Study the drawing (mm; zero at the part's minimum x, y, z) and answer. A direction names the side the tool comes from. Coordinates: 2 decimals unless noted, no trailing zeros. Write each loop counter-clockwise with the first axis right and the second up, starting at its lowest first coordinate (ties: lowest second). Pieces come first, ordered by that corner, then holes. Notation, with made-up numbers: (59, 48.5) -> (104, 48.5) arc R21 ccw to (104, 74.5) -> close; hole circle Ø4 at (41, -18). An arc over 180 degrees is marked (long way). Write each question's results on one line, items separated by ' | '. Start each with the question number.
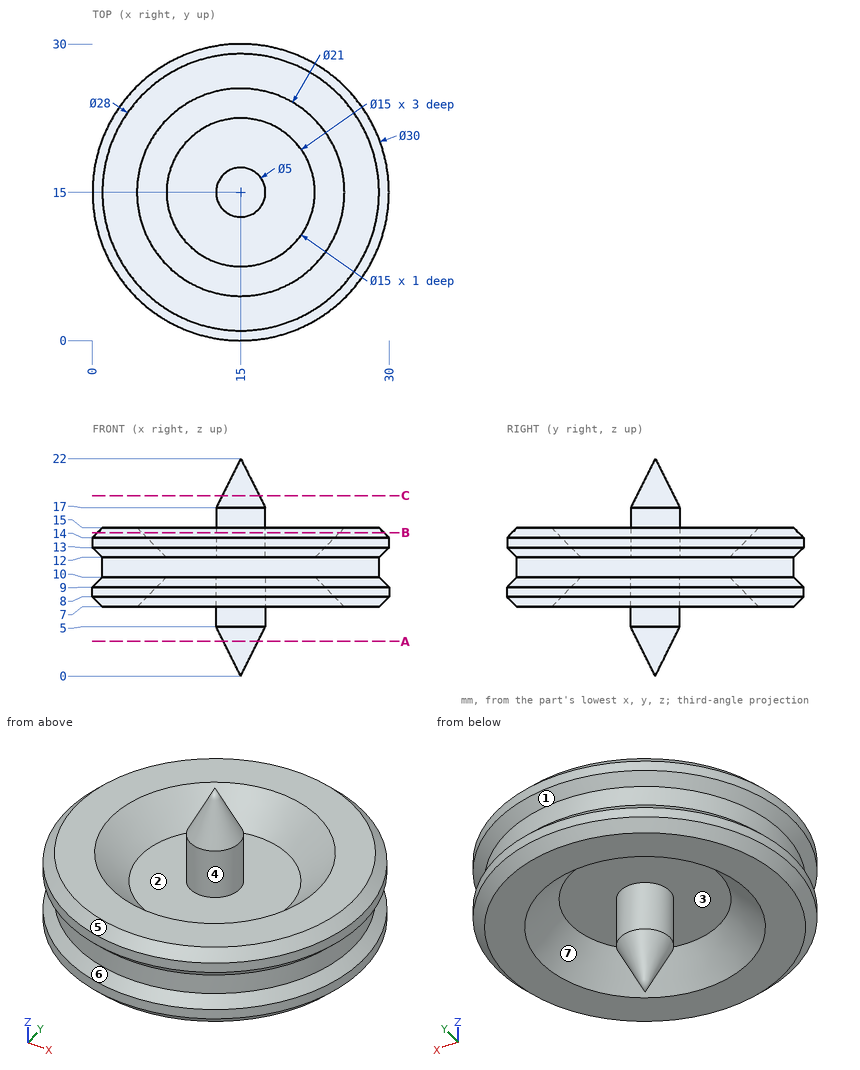
1. For the marked faces 1, 2 and 3, determine the directions among +Z, -Z, +X, -X, +Y, -Y from which every point of the face is accessible in a straight line to the end or side of a thin tool.
2. Given pin 1 Ø1.5 at (y, z) = (20.5, 14.5) entering from -X; pin 2 Ø1.5 at (x, z) = (22.5, 8) entering from -Y; pin 3 Ø1.5 at (y, z) = (14, 16.5) entering from +X, each flat-ended and moving along its own axis, determine where each tip first touches the part or whether it passes through.
3. Determine the mould class of the marked faces 4, 5, 6 and 7 for opening direction Z: pulls with the +Z half, pulls with the -Z half, needs draft (parallel to the pull), parting line crosses it, or undercut.
4. Find section A-A on z = 3.5. Give the vertices of the cut face in (x, y).
5. Find the intervals of material crossed by L1, parallel to Y at x = 15, z = 12.05; L2, parallel to Z at x = 12.75, y = 9.75; L3, parallel to Y at x = 16.75, z = 9.5, in increasing order.
6. Find section B-B on z = 14.5. Give the vertices of the cut face in (x, y), and give its area (3 significant figures).
7. Find section C-C on z = 18.25. Give the vertices of the cut face in (x, y) (3 decimals).
Ans:
1) face 1: none | face 2: +Z | face 3: -Z
2) pin 1: stops at x = 0.84 | pin 2: stops at y = 1.6 | pin 3: stops at x = 17.49
3) face 4: needs draft | face 5: pulls with the +Z half | face 6: undercut | face 7: pulls with the -Z half
4) outline: circle Ø3.5 at (15, 15)
5) L1: y = 0.95 to 7.45, 12.5 to 17.5, 22.55 to 29.05 | L2: z = 10 to 12 | L3: y = 0.61 to 7.19, 13.21 to 16.79, 22.81 to 29.39
6) outline: circle Ø29 at (15, 15); circle Ø5 at (15, 15); hole circle Ø20 at (15, 15) | area: 366 mm²
7) outline: circle Ø3.75 at (15, 15)
